from build123d import *

# Parameters (mm, degrees)
ESBO_O1_R                 = 1.6
RESSALTO_EXTRUS_O10_DEPTH = 3
FILETE2_R                 = 1
CHANFRO1_SIZE             = 1.35
ESBO_O5_W                 = 50
ESBO_O5_H                 = 13
RESSALTO_EXTRUS_O13_DEPTH = 3
ESBO_O7_R                 = 1.65
CORTE_EXTRUS_O1_DEPTH     = 4
ESBO_O8_W                 = 10
ESBO_O8_H                 = 15
CORTE_EXTRUS_O2_DEPTH     = 4
FILETE3_R                 = 3
CHANFRO2_SIZE             = 1
ESBO_O9_R                 = 4
RESSALTO_EXTRUS_O14_DEPTH = 8


with BuildPart() as part:
    # Esboço1 → Ressalto-extrusão10 (new body)
    with BuildSketch(Plane(origin=(0, 0, 0), x_dir=(1, 0, 0), z_dir=(0, 1, 0))):
        with BuildLine():
            Line((25, 20), (-25, 20))
            Line((-25, 20), (-25, -20))
            Line((-25, -20), (25, -20))
            Line((25, -20), (25, -3.31662479))
            ThreePointArc((25, -3.31662479), (14, 0), (25, 3.31662479))
            Line((25, 3.31662479), (25, 20))
        make_face()
        with Locations((20, -9)):
            Circle(ESBO_O1_R, mode=Mode.SUBTRACT)
        with Locations((20, 9)):
            Circle(ESBO_O1_R, mode=Mode.SUBTRACT)
    extrude(amount=RESSALTO_EXTRUS_O10_DEPTH)

    # Filete2
    filete2_edges = [part.edges().sort_by_distance(p)[0] for p in [
        (25, 1.5, 3.31662479),
        (25, 1.5, -3.31662479),
    ]]
    fillet(filete2_edges, radius=FILETE2_R)

    # Chanfro1
    chanfro1_edges = [part.edges().sort_by_distance(p)[0] for p in [
        (18.4, 0, -9),
        (18.4, 0, 9),
    ]]
    chamfer(chanfro1_edges, length=CHANFRO1_SIZE)

    # Esboço5 → Ressalto-extrusão13 (add)
    with BuildSketch(Plane.XZ):
        with Locations((0, 26.5)):
            Rectangle(ESBO_O5_W, ESBO_O5_H)
    extrude(amount=-RESSALTO_EXTRUS_O13_DEPTH)

    # Esboço7 → Corte-extrusão1 (cut, through all)
    with BuildSketch(Plane.XZ):
        with Locations((-15.5, 28.234562647)):
            Circle(ESBO_O7_R)
        with Locations((4.5, 28.234562647)):
            Circle(ESBO_O7_R)
    extrude(amount=-CORTE_EXTRUS_O1_DEPTH, mode=Mode.SUBTRACT)

    # Esboço8 → Corte-extrusão2 (cut, through all)
    with BuildSketch(Plane.XZ):
        Polygon((-25, -20), (-25, 13), (17, -20), align=None)
        with Locations((20, 25.5)):
            Rectangle(ESBO_O8_W, ESBO_O8_H)
    extrude(amount=-CORTE_EXTRUS_O2_DEPTH, mode=Mode.SUBTRACT)

    # Filete3
    filete3_edges = [part.edges().sort_by_distance(p)[0] for p in [
        (25, 1.5, -20),
        (-25, 1.5, 33),
        (-25, 1.5, 13),
        (17, 1.5, -20),
        (15, 1.5, 18),
        (15, 1.5, 33),
        (25, 1.5, 18),
    ]]
    fillet(filete3_edges, radius=FILETE3_R)

    # Chanfro2
    chanfro2_edges = [part.edges().sort_by_distance(p)[0] for p in [
        (-17.15, 3, 28.234562647),
        (2.85, 3, 28.234562647),
    ]]
    chamfer(chanfro2_edges, length=CHANFRO2_SIZE)

    # Esboço9 → Ressalto-extrusão14 (add)
    with BuildSketch(Plane.XZ):
        with Locations((-5.5, 10.234562647)):
            Circle(ESBO_O9_R)
    extrude(amount=RESSALTO_EXTRUS_O14_DEPTH)


solid = part.part
The listing builds one solid part. Answer for the finished solid, in the listing's coordinates (mm). A direction names the side the tool comes from. Coordinates: 2 decimals unless noted, no trailing zeros. Loops run counter-clockwise (first coordinate to the right, second up) from the corner with the lowest first, then second, coordinate; pieces in that order, holes last.
1) Find section A-A on x = 20. Write down the section's boundary in (y, z), then the cut area to 3 significant figures.
2) Find section B-B on x = -15.5. Write down the section's boundary in (y, z).
3) A tool of negligible diameter and unlimited length cuts with its end or side. For faces 5 (the face through (-5, 1, 33)), 6 (the face through (24.45, 1.52, 4.85)), 7 (the face through (-6.02, -3.94, 14.2)), 8 (the face through (20, 1, 18)), from which of +Z, -Z, +X, -X, +Y, -Y can it reach the whole face along a straight path? Write none if from no direction.
4) Find section C-C on x = -4.5. Write down the section's boundary in (y, z).
5) Find the intervals of material crossed by L1, parallel to Z at x = 20, y = 2.1; L2, parallel to X at y = 2.6, z = -9; L3, parallel to Z at x = 20, y = 0.7, in increasing order.
6) Flat-ended cylindrical pins translate along their axes: pin 1 Ø1 at (x, y) = (-8, -2.5) entering from +Z; pin 2 Ø2.5 at (x, y) = (19, 1.5) entering from +Z; pin 3 Ø4 at (x, z) = (-17, 6.5) entering from -Y. Find the tip coordinate at first contact, or state that the pin passes through.
7) Determine the mould class of faces 1 (the face through (15.86, 1.52, 18.9)), 2 (the face through (24.476, 1.521, -4.865)), 3 (the face through (-6, -8, 10)), 4 (the face through (19.65, 2.16, -7.44)) for opening direction X: pulls with the +X half, pulls with the -X half, needs draft (parallel to the pull), parting line crosses it, or undercut.
8) Find section D-D on z = 0. Write down the section's boundary in (x, y), then the cut area to 3 significant figures.
Values:
1. outline: (0, -20) - (3, -20) - (3, -10.6) - (1.35, -10.6) - (0, -11.95) - close; (0, -6.05) - (1.35, -7.4) - (3, -7.4) - (3, -6) - (0, -6) - close; (0, 6) - (3, 6) - (3, 7.4) - (1.35, 7.4) - (0, 6.05) - close; (0, 11.95) - (1.35, 10.6) - (3, 10.6) - (3, 18) - (0, 18) - close
1. area: 55.2 mm2
2. outline: (0, 5.54) - (3, 5.54) - (3, 25.58) - (2, 26.58) - (0, 26.58) - close; (0, 29.88) - (2, 29.88) - (3, 30.88) - (3, 33) - (0, 33) - close
3. face 5: +Z, +X, -X, +Y, -Y
3. face 6: +Y, -Y
3. face 7: -Y
3. face 8: +Z, +X, +Y, -Y
4. outline: (-8, 6.36) - (0, 6.36) - (0, -3.11) - (3, -3.11) - (3, 33) - (0, 33) - (0, 14.11) - (-8, 14.11) - close
5. L1: z = -20 to -10.6, -7.4 to -6, 6 to 7.4, 10.6 to 18
5. L2: x = 3 to 18.4, 21.6 to 25
5. L3: z = -20 to -11.25, -6.75 to -6, 6 to 6.75, 11.25 to 18
6. pin 1: stops at z = 13.7
6. pin 2: stops at z = 18.01
6. pin 3: stops at y = 0
7. face 1: pulls with the +X half
7. face 2: undercut
7. face 3: needs draft
7. face 4: undercut
8. outline: (-8.45, 0) - (14, 0) - (14, 3) - (-8.45, 3) - close
8. area: 67.4 mm2
